Geometry check sheet. Reference: the model listing, model coordinates, mm. Face numbers are marked on the shaded views. A direction names the side the tool comes from. Coordinates: 2 decimals unless noted, no trailing zeros. Loops run counter-clockwise (first coordinate to the right, second up) from the corner with the lowest first, then second, coordinate; pieces in that order, holes last.
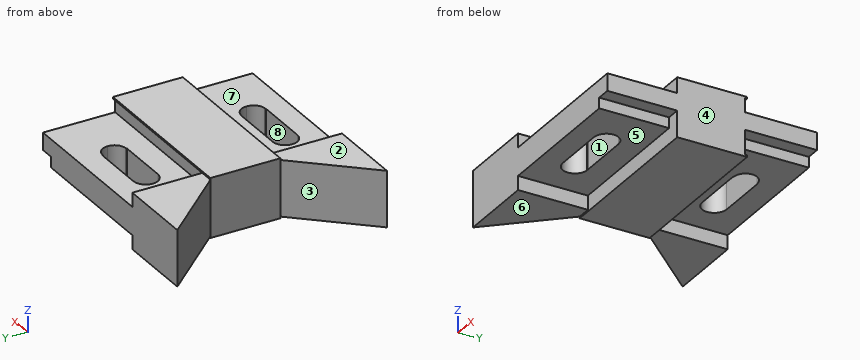
from build123d import *

# Parameters (mm, degrees)
F0_W      = 75.9690925479
F0_H      = 26.924
F1_DEPTH  = 31.75
F2_W      = 31.75
F2_H      = 25.4
F3_DEPTH  = 104.648
F4_W      = 69.596
F4_H      = 6.35
F5_DEPTH  = 32.766
F6_W      = 6.35
F6_H      = 4.826
F7_DEPTH  = 31.75
F8_DEPTH  = 31.75
F9_DEPTH  = 32.004
F10_DEPTH = 32.766
F11_DEPTH = 32.766
F12_W     = 69.596
F12_H     = 6.35
F13_DEPTH = 31.75
F14_W     = 6.35
F14_H     = 4.826
F15_DEPTH = 31.75
F17_DEPTH = 19.813
F19_DEPTH = 19.813
F21_DEPTH = 26.163
F23_DEPTH = 26.163


with BuildPart() as f1:
    # F0 (on Front) → F1 (new body)
    with BuildSketch(Plane.XZ):
        with Locations((-37.9845462739, 13.462)):
            Rectangle(F0_W, F0_H)
    extrude(amount=F1_DEPTH)

    # F2 (on face) → F3 (join)
    with BuildSketch(Plane.YZ):
        with Locations((-47.625, 13.462)):
            Rectangle(F2_W, F2_H)
        with Locations((15.875, 13.462)):
            Rectangle(F2_W, F2_H)
    extrude(amount=-F3_DEPTH)

    # F4 (on face) → F5 (cut)
    with BuildSketch(Plane(origin=(0, 31.75, 0), x_dir=(-1, 0, 0), z_dir=(0, 1, 0))):
        with Locations((34.798, 22.987)):
            Rectangle(F4_W, F4_H)
        with Locations((34.798, 3.937)):
            Rectangle(F4_W, F4_H)
    extrude(amount=-F5_DEPTH, mode=Mode.SUBTRACT)

    # F6 (on face) → F7 (join)
    with BuildSketch(Plane(origin=(0, 31.75, 0), x_dir=(-1, 0, 0), z_dir=(0, 1, 0))):
        with Locations((3.175, 9.525)):
            Rectangle(F6_W, F6_H)
    extrude(amount=-F7_DEPTH)

    # F6 (on face) → F8 (join)
    with BuildSketch(Plane(origin=(0, 31.75, 0), x_dir=(-1, 0, 0), z_dir=(0, 1, 0))):
        with Locations((3.175, 9.525)):
            Rectangle(F6_W, F6_H)
    extrude(amount=-F8_DEPTH)

    # F6 (on face) → F9 (cut)
    with BuildSketch(Plane(origin=(0, 31.75, 0), x_dir=(-1, 0, 0), z_dir=(0, 1, 0))):
        with Locations((3.175, 9.525)):
            Rectangle(F6_W, F6_H)
    extrude(amount=-F9_DEPTH, mode=Mode.SUBTRACT)

    # F6 (on face) → F10 (join)
    with BuildSketch(Plane(origin=(0, 31.75, 0), x_dir=(-1, 0, 0), z_dir=(0, 1, 0))):
        with Locations((3.175, 9.525)):
            Rectangle(F6_W, F6_H)
    extrude(amount=-F10_DEPTH)

    # F6 (on face) → F11 (cut)
    with BuildSketch(Plane(origin=(0, 31.75, 0), x_dir=(-1, 0, 0), z_dir=(0, 1, 0))):
        with Locations((3.175, 9.525)):
            Rectangle(F6_W, F6_H)
    extrude(amount=-F11_DEPTH, mode=Mode.SUBTRACT)

    # F12 (on face) → F13 (cut)
    with BuildSketch(Plane.XZ.offset(63.5)):
        with Locations((-34.798, 3.937)):
            Rectangle(F12_W, F12_H)
        with Locations((-34.798, 22.987)):
            Rectangle(F12_W, F12_H)
    extrude(amount=-F13_DEPTH, mode=Mode.SUBTRACT)

    # F14 (on face) → F15 (cut)
    with BuildSketch(Plane.XZ.offset(63.5)):
        with Locations((-3.175, 9.525)):
            Rectangle(F14_W, F14_H)
    extrude(amount=-F15_DEPTH, mode=Mode.SUBTRACT)

    # F16 (on face) → F17 (cut, through all)
    with BuildSketch(Plane.XY.offset(19.812)):
        with BuildLine():
            Line((-51.8621839583, 20.9041976536), (-51.8621839583, 9.8067118621))
            ThreePointArc((-51.8621839583, 9.8067118621), (-47.9386302296, 11.4319010292), (-46.3134410625, 15.3554547578))
            ThreePointArc((-46.3134410625, 15.3554547578), (-47.9386302296, 19.2790084865), (-51.8621839583, 20.9041976536))
        make_face()
        with BuildLine():
            ThreePointArc((-51.8621839583, 20.9041976536), (-57.410926854, 15.3554547578), (-51.8621839583, 9.8067118621))
            Line((-51.8621839583, 9.8067118621), (-51.8621839583, 20.9041976536))
        make_face()
        with BuildLine():
            Line((-51.8621839583, 9.7674547578), (-27.6167299598, 9.7674547578))
            Line((-27.6167299598, 9.7674547578), (-27.6167299598, 10.0103156582))
            ThreePointArc((-27.6167299598, 10.0103156582), (-32.9618690595, 15.3554547578), (-27.6167299598, 20.7005938574))
            Line((-27.6167299598, 20.7005938574), (-27.6167299598, 20.9434547578))
            Line((-27.6167299598, 20.9434547578), (-51.8621839583, 20.9434547578))
            Line((-51.8621839583, 20.9434547578), (-51.8621839583, 20.9041976536))
            ThreePointArc((-51.8621839583, 20.9041976536), (-47.9386302296, 19.2790084865), (-46.3134410625, 15.3554547578))
            ThreePointArc((-46.3134410625, 15.3554547578), (-47.9386302296, 11.4319010292), (-51.8621839583, 9.8067118621))
            Line((-51.8621839583, 9.8067118621), (-51.8621839583, 9.7674547578))
        make_face()
        with BuildLine():
            ThreePointArc((-27.6167299598, 20.7005938574), (-32.9618690595, 15.3554547578), (-27.6167299598, 10.0103156582))
            Line((-27.6167299598, 10.0103156582), (-27.6167299598, 20.7005938574))
        make_face()
        with BuildLine():
            Line((-27.6167299598, 20.7005938574), (-27.6167299598, 10.0103156582))
            ThreePointArc((-27.6167299598, 10.0103156582), (-23.8371458561, 11.5758706541), (-22.2715908602, 15.3554547578))
            ThreePointArc((-22.2715908602, 15.3554547578), (-23.8371458561, 19.1350388615), (-27.6167299598, 20.7005938574))
        make_face()
    extrude(amount=-F17_DEPTH, mode=Mode.SUBTRACT)

    # F18 (on face) → F19 (cut, through all)
    with BuildSketch(Plane.XY.offset(19.812)):
        with BuildLine():
            Line((-51.8621839583, -53.5478262464), (-27.3858178407, -53.5478262464))
            Line((-27.3858178407, -53.5478262464), (-27.3858178407, -53.4538679724))
            ThreePointArc((-27.3858178407, -53.4538679724), (-32.8798595667, -47.9598262464), (-27.3858178407, -42.4657845204))
            Line((-27.3858178407, -42.4657845204), (-27.3858178407, -42.3718262464))
            Line((-27.3858178407, -42.3718262464), (-51.8621839583, -42.3718262464))
            Line((-51.8621839583, -42.3718262464), (-51.8621839583, -42.3927269235))
            ThreePointArc((-51.8621839583, -42.3927269235), (-47.9256502755, -44.0232925636), (-46.2950846354, -47.9598262464))
            ThreePointArc((-46.2950846354, -47.9598262464), (-47.9256502755, -51.8963599291), (-51.8621839583, -53.5269255693))
            Line((-51.8621839583, -53.5269255693), (-51.8621839583, -53.5478262464))
        make_face()
        with BuildLine():
            ThreePointArc((-27.3858178407, -42.4657845204), (-32.8798595667, -47.9598262464), (-27.3858178407, -53.4538679724))
            Line((-27.3858178407, -53.4538679724), (-27.3858178407, -42.4657845204))
        make_face()
        with BuildLine():
            Line((-27.3858178407, -42.4657845204), (-27.3858178407, -53.4538679724))
            ThreePointArc((-27.3858178407, -53.4538679724), (-23.5009436801, -51.844700407), (-21.8917761147, -47.9598262464))
            ThreePointArc((-21.8917761147, -47.9598262464), (-23.5009436801, -44.0749520858), (-27.3858178407, -42.4657845204))
        make_face()
        with BuildLine():
            ThreePointArc((-51.8621839583, -42.3927269235), (-57.4292832812, -47.9598262464), (-51.8621839583, -53.5269255693))
            Line((-51.8621839583, -53.5269255693), (-51.8621839583, -42.3927269235))
        make_face()
        with BuildLine():
            Line((-51.8621839583, -42.3927269235), (-51.8621839583, -53.5269255693))
            ThreePointArc((-51.8621839583, -53.5269255693), (-47.9256502755, -51.8963599291), (-46.2950846354, -47.9598262464))
            ThreePointArc((-46.2950846354, -47.9598262464), (-47.9256502755, -44.0232925636), (-51.8621839583, -42.3927269235))
        make_face()
    extrude(amount=-F19_DEPTH, mode=Mode.SUBTRACT)

    # F20 (on face) → F21 (cut, through all)
    with BuildSketch(Plane.XY.offset(26.162)):
        Polygon((-104.648, -31.75), (-104.648, -63.5), (-75.9690925479, -31.75), align=None)
    extrude(amount=-F21_DEPTH, mode=Mode.SUBTRACT)

    # F22 (on face) → F23 (cut, through all)
    with BuildSketch(Plane.XY.offset(26.162)):
        Polygon((-104.648, 0), (-75.9690925479, 0), (-104.648, 31.75), align=None)
    extrude(amount=-F23_DEPTH, mode=Mode.SUBTRACT)


solid = f1.part
(1) Access from +Z, -Z, +X, -X, +Y, -Y to the whole of each face (thin tool, end or side, straight path). Record for the marked faces 5, 6, 7 and 8.
Findings:
face 5: -Z, +X, -Y
face 6: -Z, +X, -X, -Y
face 7: +Z, +X, -Y
face 8: +Z, -Z
(2) Sectioned sample at A-A on z = 18.25. State how many separate pieces and enclosed holes the cut face has, and give its area (3 significant figures).
Findings:
separate pieces: 1
enclosed holes: 2
area: 7,410 mm2
(3) Sectioned sample at D-D on x = -71.5. Record the cut outline in (y, z), and give its area (3 significant figures).
Findings:
outline: (-63.5, 0.76) - (-31.75, 0.76) - (-31.75, 0) - (0, 0) - (0, 0.76) - (31.75, 0.76) - (31.75, 26.16) - (0, 26.16) - (0, 26.92) - (-31.75, 26.92) - (-31.75, 26.16) - (-63.5, 26.16) - close
area: 2,470 mm2
(4) Draft check along X on the marked faces 1, 2, 3 and 4. Enter one of: +X half, -X half, draft (parallel to the pull), parting line (faces both ways), or undercut.
Findings:
face 1: undercut
face 2: draft
face 3: -X half
face 4: +X half
(5) Sectioned sample at C-C on y = -52. Record the cut outline in (x, z), and give its area (3 significant figures).
Findings:
outline: (-94.26, 0.76) - (-69.6, 0.76) - (-69.6, 7.11) - (-55.69, 7.11) - (-55.69, 19.81) - (-69.6, 19.81) - (-69.6, 26.16) - (-94.26, 26.16) - close; (-23.66, 7.11) - (-6.35, 7.11) - (-6.35, 11.94) - (0, 11.94) - (0, 19.81) - (-23.66, 19.81) - close
area: 1,070 mm2
(6) Scan lines: L1, parallel to Y at x = -43.5, z = 15.25; L2, parallel to Z at x = -62, y = -0.5; L3, parallel to X at y = -11.5, z = 14.5. Record each from-to range of solid material in increasing order.
Findings:
L1: y = -63.5 to -53.55, -42.37 to 9.77, 20.94 to 31.75
L2: z = 0 to 0.76, 7.11 to 19.81, 26.16 to 26.92
L3: x = -75.97 to 0
(7) Gauge pin test, flat ends, axial feed: pin 1 Ø2.5 at (y, z) = (-53, 10.5) entering from +X; pin 2 Ø7 at (y, z) = (11.5, 3) entering from +X; pin 3 Ø1.5 at (x, y) = (-16, 20) entering from -Z. Record the tip position at first contact, or that the pin passes through.
Findings:
pin 1: stops at x = -6.35
pin 2: stops at x = -69.6
pin 3: stops at z = 7.11
(8) Sectioned sample at B-B on x = -31. Record the cut outline in (y, z).
Findings:
outline: (-63.5, 7.11) - (-53.55, 7.11) - (-53.55, 19.81) - (-63.5, 19.81) - close; (-42.37, 7.11) - (-31.75, 7.11) - (-31.75, 0) - (0, 0) - (0, 0.76) - (-1.02, 0.76) - (-1.02, 7.11) - (9.77, 7.11) - (9.77, 19.81) - (-1.02, 19.81) - (-1.02, 26.16) - (0, 26.16) - (0, 26.92) - (-31.75, 26.92) - (-31.75, 19.81) - (-42.37, 19.81) - close; (20.94, 7.11) - (31.75, 7.11) - (31.75, 19.81) - (20.94, 19.81) - close
